Source: CAD feature listing. Evaluate the final solid. Frame: model axes, mm. A direction names the side the tool comes from. Give positions to 0.01 mm unless a question says otherwise; leave off trailing zeros. Loops run counter-clockwise (first coordinate to the right, second up) from the corner with the lowest first, then second, coordinate; pieces in that order, holes last. Notation, with made-up numbers: (8, 2) - (61, 2) arc R12 cw to (61, 18) - close; hole circle Ø1 at (31, 17). An arc over 180 degrees is marked (long way). Put each result on its own line as item: value.
Autodesk Inventor part; units mm, degrees
ref_plane "YZ Plane" through (0, 0, 0) normal (1, 0, 0) x (0, 1, 0)
ref_plane "XZ Plane" through (0, 0, 0) normal (0, 1, 0) x (-1, 0, 0)
ref_plane "XY Plane" through (0, 0, 0) normal (0, 0, 1) x (1, 0, 0)
sketch "スケッチ1" plane through (0, 0, 0) normal (0, 0, 1) x (1, 0, 0)
  circle A0 centre (0, 0) radius 5.15
  dimension "d0" = 10.3
extrude "押し出し1" add sketch "スケッチ1" along normal blind 1.75
sketch "スケッチ2" plane through (0, 0, 1.75) normal (0, 0, 1) x (1, 0, 0)
  circle A0 centre (0, 0) radius 4.5
  dimension "d3" = 9
extrude "押し出し2" add sketch "スケッチ2" along normal blind 7
thread "ねじ1"
sketch "スケッチ3" plane through (0, 0, 8.75) normal (0, 0, 1) x (1, 0, 0)
  circle A0 centre (0, 0) radius 3
  dimension "d8" = 6
extrude "押し出し3" add sketch "スケッチ3" along normal blind 12
sketch "スケッチ4" plane through (0, 0, 0) normal (0, 0, -1) x (-1, 0, 0)
  circle A0 centre (0, 0) radius 11.175
  dimension "d11" = 22.35
extrude "押し出し4" add sketch "スケッチ4" along normal blind 20
properties part number "ポテンショメータB"
1) Section query B-B, the plane x = -1.5. Output: boundary loops of the cut face in (y, z), plus the area to 3 significant figures.
Check result:
outline: (-11.07, -20) - (11.07, -20) - (11.07, 0) - (4.93, 0) - (4.93, 1.75) - (4.24, 1.75) - (4.24, 8.75) - (2.6, 8.75) - (2.6, 20.75) - (-2.6, 20.75) - (-2.6, 8.75) - (-4.24, 8.75) - (-4.24, 1.75) - (-4.93, 1.75) - (-4.93, 0) - (-11.07, 0) - close
area: 582 mm²
2) Section query A-A, the plane y = 0. Output: boundary loops of the cut face in (x, z) (3 decimals).
Check result:
outline: (-11.175, -20) - (11.175, -20) - (11.175, 0) - (5.15, 0) - (5.15, 1.75) - (4.5, 1.75) - (4.5, 8.75) - (3, 8.75) - (3, 20.75) - (-3, 20.75) - (-3, 8.75) - (-4.5, 8.75) - (-4.5, 1.75) - (-5.15, 1.75) - (-5.15, 0) - (-11.175, 0) - close
3) Access query for faces 1 (the flat face through (0, 0, 20.75)), 2 (the flat face through (0, -5, 1.75)). Directions: +Z, -Z, +X, -X, +Y, -Y. A direction counts if a zero-diameter tool reaches every point of the face in a straight line with its end or side. Return the directions, or none.
Check result:
face 1: +Z, +X, -X, +Y, -Y
face 2: +Z
4) Pin query (flat end, axial travel): P1, Ø8, axis at y = -8, z = 1, coming from the -X side (3 decimals); P2, Ø2, axis at y = -6, z = -4, coming from the -X side; P3, Ø12, axis at y = 6, z = 15.5, coming from the +X side; P4, Ø2, axis at x = 4.5, z = 10.5, coming from the -Y side. Return the tip coordinate at first contact, or that it passes through.
Check result:
P1: x = -10.385
P2: x = -9.99
P3: x = 3
P4: through
5) Material intervals for line 1 along Z through (x, y) = (-2.75, -3); line 2 along Y through (x, z) = (0, 16); line 3 along Z through (x, y) = (-8.75, 1), sorted ascending. Write a range as [from, to].
Check result:
line 1: [-20, 8.75]
line 2: [-3, 3]
line 3: [-20, 0]
6) Section query C-C, the plane z = -7.5. Output: boundary loops of the cut face in (x, y) (3 decimals), plus the area to 3 significant figures.
Check result:
outline: circle Ø22.35 at (0, 0)
area: 392 mm²
7) Section query D-D, the plane z = 5. Output: boundary loops of the cut face in (x, y).
Check result:
outline: circle Ø9 at (0, 0)
